from build123d import *

# Parameters (mm, degrees)
F0_W     = 705.358
F0_H     = 88.9
F1_DEPTH = 44.45
F4_W     = 88.9
F4_H     = 88.9
F4_W_2   = 38.1
F4_H_2   = 50.8
F5_REACH = 193.287585695
F6_W     = 88.9
F6_H     = 88.9
F6_W_2   = 38.1
F6_H_2   = 50.8
F7_DEPTH = 38.1
F9_DEPTH = 88.901


with BuildPart() as f1:
    # F0 (on Right) → F1 (new body, symmetric)
    with BuildSketch(Plane.YZ):
        Rectangle(F0_W, F0_H)
    extrude(amount=F1_DEPTH, both=True)

    f5_end = Plane(origin=(0, 233.0836645991, 134.5709165), x_dir=(0, -0.5, 0.8660254038), z_dir=(0, 0.8660254038, 0.5))
    # F4 (on face) → F5 (cut, up to a plane its end follows)
    with BuildSketch(Plane(origin=(0, 352.679, 0), x_dir=(-1, 0, 0), z_dir=(0, 1, 0))):
        Rectangle(F4_W, F4_H)
        Rectangle(F4_W_2, F4_H_2, mode=Mode.SUBTRACT)
    f5_long = extrude(amount=-F5_REACH, mode=Mode.PRIVATE)
    add(split(f5_long, bisect_by=f5_end, keep=Keep.TOP, mode=Mode.PRIVATE), mode=Mode.SUBTRACT)

    # F6 (on face) → F7 (cut)
    with BuildSketch(Plane.XZ.offset(352.679)):
        Rectangle(F6_W, F6_H)
        Rectangle(F6_W_2, F6_H_2, mode=Mode.SUBTRACT)
    extrude(amount=-F7_DEPTH, mode=Mode.SUBTRACT)

    # F8 (on face) → F9 (cut, through all)
    with BuildSketch(Plane.YZ.offset(44.45)):
        Polygon((-35.179, -6.35), (-35.179, 6.35), (-238.379, 6.35), (-238.379, -6.35), (-200.279, -6.35), (-200.279, -25.4), (-181.229, -25.4), (-181.229, -6.35), (-92.329, -6.35), (-92.329, -25.4), (-73.279, -25.4), (-73.279, -6.35), align=None)
    extrude(amount=-F9_DEPTH, mode=Mode.SUBTRACT)


solid = f1.part
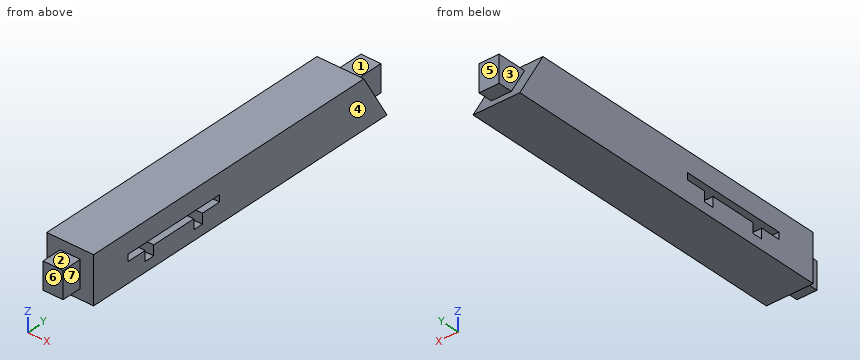
Design review of the part built by this model. Coordinates are the model's own, in mm. Face numbers are marked on the shaded views. A direction names the side the tool comes from. Round coordinates to 2 decimals unless told otherwise and drop trailing zeros. Write each loop counter-clockwise with the first axis right and the second up, starting at its lowest first coordinate (ties: lowest second). Pieces come first, ordered by that corner, then holes. Notation, with made-up numbers: (-36, -18.5) -> (14, -18.5) arc R19 cw to (14, -13.5) -> close; hole circle Ø9 at (65, 14). An arc over 180 degrees is marked (long way). One line per item, written item: value. Start each with the question number.
Q1. Add section A-A (x = -33.5). Give the boundary of the cut face in (y, z) (3 decimals), then the cut area to 3 significant figures.
Q2. Add section C-C (z = -18). Give the boundary of the cut face in (x, y), then the cut area to 3 significant figures.
Q3. Tool access review of the marked faces 1, 2, 3 and 4: name each direction out of +Z, -Z, +X, -X, +Y, -Y from which nothing blocks a thin tool from reaching the whole face with its end or side.
Q4. To check wall thickness, follow probe 1 along Y at (x, z) = (9, -6.5); probe 2 along Y at (x, z) = (5, -4); probe 3 along Z at (x, y) = (10, -42). State the ranges of each line that lie inside material, in increasing order.
Q5. Insertion check: P1, Ø1.5, axis at x = 30.5, z = -0.5, coming from the -Y side; P2, Ø19, axis at x = -2.5, y = -330, coming from the -Z side; P3, Ø11.5, axis at x = 2, y = -341.5, coming from the +Z side. Each pin has a flat end and moves straight along its axis. Give the tip position at first contact, or say it passes through.
Q6. The part is to be moulded in two halves that separate along Y. For the marked faces 5, 6 and 7, say which applies: pulls with the +Y half, pulls with the -Y half, needs draft (parallel to the pull), parting line crosses it, or undercut.
Q7. Add section B-B (y = -165). Give the boundary of the cut face in (x, z), then the cut area to 3 significant figures.
Q8. Add section D-D (x = 7.5). Give the boundary of the cut face in (y, z) (3 decimals).
Response:
1. outline: (-314.579, -44.45) -> (336.441, -44.45) -> (285.115, 44.45) -> (-314.579, 44.45) -> close; hole (-238.379, -6.35) -> (-200.279, -6.35) -> (-200.279, -25.4) -> (-181.229, -25.4) -> (-181.229, -6.35) -> (-92.329, -6.35) -> (-92.329, -25.4) -> (-73.279, -25.4) -> (-73.279, -6.35) -> (-35.179, -6.35) -> (-35.179, 6.35) -> (-238.379, 6.35) -> close
1. area: 52,300 mm^2
2. outline: (-44.45, -314.58) -> (-19.05, -314.58) -> (-19.05, -352.68) -> (19.05, -352.68) -> (19.05, -314.58) -> (44.45, -314.58) -> (44.45, -200.28) -> (-44.45, -200.28) -> close; (-44.45, -181.23) -> (44.45, -181.23) -> (44.45, -92.33) -> (-44.45, -92.33) -> close; (-44.45, -73.28) -> (44.45, -73.28) -> (44.45, 321.17) -> (19.05, 321.17) -> (19.05, 352.68) -> (-19.05, 352.68) -> (-19.05, 321.17) -> (-44.45, 321.17) -> close
2. area: 55,800 mm^2
3. face 1: +Z, +X, -X, +Y
3. face 2: +Z, +X, -X, -Y
3. face 3: +Z, -X, +Y
3. face 4: +Z, -Z, +X, +Y, -Y
4. probe 1: y = -352.68 to -200.28, -181.23 to -92.33, -73.28 to 352.68
4. probe 2: y = -352.68 to -238.38, -35.18 to 352.68
4. probe 3: z = -44.45 to -6.35, 6.35 to 44.45
5. P1: stops at y = -314.58
5. P2: stops at z = -25.4
5. P3: stops at z = 25.4
6. face 5: pulls with the +Y half
6. face 6: pulls with the -Y half
6. face 7: needs draft
7. outline: (-44.45, -44.45) -> (44.45, -44.45) -> (44.45, -6.35) -> (-44.45, -6.35) -> close; (-44.45, 6.35) -> (44.45, 6.35) -> (44.45, 44.45) -> (-44.45, 44.45) -> close
7. area: 6,770 mm^2
8. outline: (-352.679, -25.4) -> (-314.579, -25.4) -> (-314.579, -44.45) -> (336.441, -44.45) -> (325.443, -25.4) -> (352.679, -25.4) -> (352.679, 25.4) -> (296.114, 25.4) -> (285.115, 44.45) -> (-314.579, 44.45) -> (-314.579, 25.4) -> (-352.679, 25.4) -> close; hole (-238.379, -6.35) -> (-200.279, -6.35) -> (-200.279, -25.4) -> (-181.229, -25.4) -> (-181.229, -6.35) -> (-92.329, -6.35) -> (-92.329, -25.4) -> (-73.279, -25.4) -> (-73.279, -6.35) -> (-35.179, -6.35) -> (-35.179, 6.35) -> (-238.379, 6.35) -> close
